Part model, mm, in its own coordinate system. Give positions to 0.01 mm unless a question says otherwise; leave off trailing zeros. Write each loop counter-clockwise with the first axis right and the second up, starting at its lowest first coordinate (ties: lowest second). Pieces come first, ordered by that corner, then holes. Notation, with made-up numbers: (80, 53) - (109, 53) arc R10 ccw to (109, 61) - close; hole circle Ø1 at (53.25, 29.25). An arc over 180 degrees is marked (long way). Answer as a JSON object with one key per item and string values. Group by question number.
```python
from build123d import *

# Parameters (mm, degrees)
BOSS_EXTRUDE1_DEPTH          = 3
MOUNTING_SLOTS_REACH         = 173.039
SKETCH2_W                    = 3.2
SKETCH2_H                    = 15
CASTER_AND_WHEEL_SLOTS_REACH = 173.039
SKETCH3_R                    = 4.7
SKETCH3_W                    = 12
SKETCH3_H                    = 68


with BuildPart() as part:
    # Sketch1 → Boss-Extrude1 (new body)
    with BuildSketch(Plane.XY):
        with BuildLine():
            Line((-107.5, -45.307284183), (-107.5, 47.371965948))
            ThreePointArc((-107.5, 47.371965948), (-94.261836832, 91.449819149), (-58.928571429, 120.939927031))
            ThreePointArc((-58.928571429, 120.939927031), (0, 133), (58.928571429, 120.939927031))
            ThreePointArc((58.928571429, 120.939927031), (94.261836832, 91.449819149), (107.5, 47.371965948))
            Line((107.5, 47.371965948), (107.5, -45.307284183))
            ThreePointArc((107.5, -45.307284183), (97.216406667, -84.545309636), (69.009433962, -113.695637666))
            ThreePointArc((69.009433962, -113.695637666), (0, -133), (-69.009433962, -113.695637666))
            ThreePointArc((-69.009433962, -113.695637666), (-97.216406667, -84.545309636), (-107.5, -45.307284183))
        make_face()
    extrude(amount=BOSS_EXTRUDE1_DEPTH)

    # Sketch2 → mounting slots (cut, up to next)
    with BuildSketch(Plane.XY.offset(3), mode=Mode.PRIVATE) as mounting_slots_sk1:
        with Locations((98.1, -52.5)):
            Rectangle(SKETCH2_W, SKETCH2_H)
    mounting_slots_tool1 = extrude(mounting_slots_sk1.sketch, amount=-MOUNTING_SLOTS_REACH, mode=Mode.PRIVATE) & part.part
    # Sketch2 → mounting slots (cut, up to next)
    with BuildSketch(Plane.XY.offset(3), mode=Mode.PRIVATE) as mounting_slots_sk2:
        with Locations((98.1, 52.5)):
            Rectangle(SKETCH2_W, SKETCH2_H)
    mounting_slots_tool2 = extrude(mounting_slots_sk2.sketch, amount=-MOUNTING_SLOTS_REACH, mode=Mode.PRIVATE) & part.part
    # Sketch2 → mounting slots (cut, up to next)
    with BuildSketch(Plane.XY.offset(3), mode=Mode.PRIVATE) as mounting_slots_sk3:
        with Locations((-98.1, 52.5)):
            Rectangle(SKETCH2_W, SKETCH2_H)
    mounting_slots_tool3 = extrude(mounting_slots_sk3.sketch, amount=-MOUNTING_SLOTS_REACH, mode=Mode.PRIVATE) & part.part
    # Sketch2 → mounting slots (cut, up to next)
    with BuildSketch(Plane.XY.offset(3), mode=Mode.PRIVATE) as mounting_slots_sk4:
        with Locations((-98.1, -52.5)):
            Rectangle(SKETCH2_W, SKETCH2_H)
    mounting_slots_tool4 = extrude(mounting_slots_sk4.sketch, amount=-MOUNTING_SLOTS_REACH, mode=Mode.PRIVATE) & part.part
    # Sketch2 → mounting slots (cut, up to next)
    with BuildSketch(Plane.XY.offset(3), mode=Mode.PRIVATE) as mounting_slots_sk5:
        with Locations((52.79, 97.254160418)):
            Rectangle(SKETCH2_W, SKETCH2_H)
    mounting_slots_tool5 = extrude(mounting_slots_sk5.sketch, amount=-MOUNTING_SLOTS_REACH, mode=Mode.PRIVATE) & part.part
    # Sketch2 → mounting slots (cut, up to next)
    with BuildSketch(Plane.XY.offset(3), mode=Mode.PRIVATE) as mounting_slots_sk6:
        with Locations((52.79, -97.254160418)):
            Rectangle(SKETCH2_W, SKETCH2_H)
    mounting_slots_tool6 = extrude(mounting_slots_sk6.sketch, amount=-MOUNTING_SLOTS_REACH, mode=Mode.PRIVATE) & part.part
    # Sketch2 → mounting slots (cut, up to next)
    with BuildSketch(Plane.XY.offset(3), mode=Mode.PRIVATE) as mounting_slots_sk7:
        with Locations((-52.79, 97.254160418)):
            Rectangle(SKETCH2_W, SKETCH2_H)
    mounting_slots_tool7 = extrude(mounting_slots_sk7.sketch, amount=-MOUNTING_SLOTS_REACH, mode=Mode.PRIVATE) & part.part
    # Sketch2 → mounting slots (cut, up to next)
    with BuildSketch(Plane.XY.offset(3), mode=Mode.PRIVATE) as mounting_slots_sk8:
        with Locations((-52.79, -97.254160418)):
            Rectangle(SKETCH2_W, SKETCH2_H)
    mounting_slots_tool8 = extrude(mounting_slots_sk8.sketch, amount=-MOUNTING_SLOTS_REACH, mode=Mode.PRIVATE) & part.part
    # Sketch2 → mounting slots (cut, up to next)
    with BuildSketch(Plane.XY.offset(3), mode=Mode.PRIVATE) as mounting_slots_sk9:
        with BuildLine():
            Line((31.1, -18.6), (61.1, -18.6))
            Line((61.1, -18.6), (61.1, -15.1))
            Line((61.1, -15.1), (53.5, -15.1))
            Line((53.5, -15.1), (53, -13.6))
            Line((53, -13.6), (53.5, -13.6))
            Line((53.5, -13.6), (53.5, -10.5))
            Line((53.5, -10.5), (40.7, -10.5))
            Line((40.7, -10.5), (40.7, -7.6))
            ThreePointArc((40.7, -7.6), (39.7, -6.6), (38.7, -7.6))
            Line((38.7, -7.6), (38.7, -10.5))
            Line((38.7, -10.5), (38.9, -13.6))
            Line((38.9, -13.6), (39.4, -13.6))
            Line((39.4, -13.6), (38.9, -15.1))
            Line((38.9, -15.1), (36.2, -15.1))
            Line((36.2, -15.1), (36.2, -7.6))
            ThreePointArc((36.2, -7.6), (35.2, -6.6), (34.2, -7.6))
            Line((34.2, -7.6), (34.2, -15.1))
            Line((34.2, -15.1), (31.1, -15.1))
            Line((31.1, -15.1), (31.1, -18.6))
        make_face()
    mounting_slots_tool9 = extrude(mounting_slots_sk9.sketch, amount=-MOUNTING_SLOTS_REACH, mode=Mode.PRIVATE) & part.part
    # Sketch2 → mounting slots (cut, up to next)
    with BuildSketch(Plane.XY.offset(3), mode=Mode.PRIVATE) as mounting_slots_sk10:
        with BuildLine():
            Line((31.1, 5.4), (61.1, 5.4))
            Line((61.1, 5.4), (61.1, 8.9))
            Line((61.1, 8.9), (53.5, 8.9))
            Line((53.5, 8.9), (53, 10.4))
            Line((53, 10.4), (53.5, 10.4))
            Line((53.5, 10.4), (53.5, 13.5))
            Line((53.5, 13.5), (40.7, 13.5))
            Line((40.7, 13.5), (40.7, 16.4))
            ThreePointArc((40.7, 16.4), (39.7, 17.4), (38.7, 16.4))
            Line((38.7, 16.4), (38.7, 13.5))
            Line((38.7, 13.5), (38.9, 10.4))
            Line((38.9, 10.4), (39.4, 10.4))
            Line((39.4, 10.4), (38.9, 8.9))
            Line((38.9, 8.9), (36.2, 8.9))
            Line((36.2, 8.9), (36.2, 16.4))
            ThreePointArc((36.2, 16.4), (35.2, 17.4), (34.2, 16.4))
            Line((34.2, 16.4), (34.2, 8.9))
            Line((34.2, 8.9), (31.1, 8.9))
            Line((31.1, 8.9), (31.1, 5.4))
        make_face()
    mounting_slots_tool10 = extrude(mounting_slots_sk10.sketch, amount=-MOUNTING_SLOTS_REACH, mode=Mode.PRIVATE) & part.part
    # Sketch2 → mounting slots (cut, up to next)
    with BuildSketch(Plane.XY.offset(3), mode=Mode.PRIVATE) as mounting_slots_sk11:
        with BuildLine():
            Line((-60.9, -18.6), (-30.9, -18.6))
            Line((-30.9, -18.6), (-30.9, -15.1))
            Line((-30.9, -15.1), (-38.5, -15.1))
            Line((-38.5, -15.1), (-39, -13.6))
            Line((-39, -13.6), (-38.5, -13.6))
            Line((-38.5, -13.6), (-38.5, -10.5))
            Line((-38.5, -10.5), (-51.3, -10.5))
            Line((-51.3, -10.5), (-51.3, -7.6))
            ThreePointArc((-51.3, -7.6), (-52.3, -6.6), (-53.3, -7.6))
            Line((-53.3, -7.6), (-53.3, -10.5))
            Line((-53.3, -10.5), (-53.1, -13.6))
            Line((-53.1, -13.6), (-52.6, -13.6))
            Line((-52.6, -13.6), (-53.1, -15.1))
            Line((-53.1, -15.1), (-55.8, -15.1))
            Line((-55.8, -15.1), (-55.8, -7.6))
            ThreePointArc((-55.8, -7.6), (-56.8, -6.6), (-57.8, -7.6))
            Line((-57.8, -7.6), (-57.8, -15.1))
            Line((-57.8, -15.1), (-60.9, -15.1))
            Line((-60.9, -15.1), (-60.9, -18.6))
        make_face()
    mounting_slots_tool11 = extrude(mounting_slots_sk11.sketch, amount=-MOUNTING_SLOTS_REACH, mode=Mode.PRIVATE) & part.part
    # Sketch2 → mounting slots (cut, up to next)
    with BuildSketch(Plane.XY.offset(3), mode=Mode.PRIVATE) as mounting_slots_sk12:
        with BuildLine():
            Line((-60.9, 5.4), (-30.9, 5.4))
            Line((-30.9, 5.4), (-30.9, 8.9))
            Line((-30.9, 8.9), (-38.5, 8.9))
            Line((-38.5, 8.9), (-39, 10.4))
            Line((-39, 10.4), (-38.5, 10.4))
            Line((-38.5, 10.4), (-38.5, 13.5))
            Line((-38.5, 13.5), (-51.3, 13.5))
            Line((-51.3, 13.5), (-51.3, 16.4))
            ThreePointArc((-51.3, 16.4), (-52.3, 17.4), (-53.3, 16.4))
            Line((-53.3, 16.4), (-53.3, 13.5))
            Line((-53.3, 13.5), (-53.1, 10.4))
            Line((-53.1, 10.4), (-52.6, 10.4))
            Line((-52.6, 10.4), (-53.1, 8.9))
            Line((-53.1, 8.9), (-55.8, 8.9))
            Line((-55.8, 8.9), (-55.8, 16.4))
            ThreePointArc((-55.8, 16.4), (-56.8, 17.4), (-57.8, 16.4))
            Line((-57.8, 16.4), (-57.8, 8.9))
            Line((-57.8, 8.9), (-60.9, 8.9))
            Line((-60.9, 8.9), (-60.9, 5.4))
        make_face()
    mounting_slots_tool12 = extrude(mounting_slots_sk12.sketch, amount=-MOUNTING_SLOTS_REACH, mode=Mode.PRIVATE) & part.part
    add(mounting_slots_tool1.solids().sort_by_distance((98.1, -52.5, 3))[0], mode=Mode.SUBTRACT)
    add(mounting_slots_tool2.solids().sort_by_distance((98.1, 52.5, 3))[0], mode=Mode.SUBTRACT)
    add(mounting_slots_tool3.solids().sort_by_distance((-98.1, 52.5, 3))[0], mode=Mode.SUBTRACT)
    add(mounting_slots_tool4.solids().sort_by_distance((-98.1, -52.5, 3))[0], mode=Mode.SUBTRACT)
    add(mounting_slots_tool5.solids().sort_by_distance((52.79, 97.25416, 3))[0], mode=Mode.SUBTRACT)
    add(mounting_slots_tool6.solids().sort_by_distance((52.79, -97.25416, 3))[0], mode=Mode.SUBTRACT)
    add(mounting_slots_tool7.solids().sort_by_distance((-52.79, 97.25416, 3))[0], mode=Mode.SUBTRACT)
    add(mounting_slots_tool8.solids().sort_by_distance((-52.79, -97.25416, 3))[0], mode=Mode.SUBTRACT)
    add(mounting_slots_tool9.solids().sort_by_distance((44.9582, -14.653776, 3))[0], mode=Mode.SUBTRACT)
    add(mounting_slots_tool10.solids().sort_by_distance((44.9582, 9.346224, 3))[0], mode=Mode.SUBTRACT)
    add(mounting_slots_tool11.solids().sort_by_distance((-47.0418, -14.653776, 3))[0], mode=Mode.SUBTRACT)
    add(mounting_slots_tool12.solids().sort_by_distance((-47.0418, 9.346224, 3))[0], mode=Mode.SUBTRACT)

    # Sketch3 → caster and wheel slots (cut, up to next)
    with BuildSketch(Plane.XY.offset(3), mode=Mode.PRIVATE) as caster_and_wheel_slots_sk1:
        with Locations((0, 118)):
            Circle(SKETCH3_R)
    caster_and_wheel_slots_tool1 = extrude(caster_and_wheel_slots_sk1.sketch, amount=-CASTER_AND_WHEEL_SLOTS_REACH, mode=Mode.PRIVATE) & part.part
    # Sketch3 → caster and wheel slots (cut, up to next)
    with BuildSketch(Plane.XY.offset(3), mode=Mode.PRIVATE) as caster_and_wheel_slots_sk2:
        with Locations((75, -46)):
            Rectangle(SKETCH3_W, SKETCH3_H)
    caster_and_wheel_slots_tool2 = extrude(caster_and_wheel_slots_sk2.sketch, amount=-CASTER_AND_WHEEL_SLOTS_REACH, mode=Mode.PRIVATE) & part.part
    # Sketch3 → caster and wheel slots (cut, up to next)
    with BuildSketch(Plane.XY.offset(3), mode=Mode.PRIVATE) as caster_and_wheel_slots_sk3:
        with Locations((-75, -46)):
            Rectangle(SKETCH3_W, SKETCH3_H)
    caster_and_wheel_slots_tool3 = extrude(caster_and_wheel_slots_sk3.sketch, amount=-CASTER_AND_WHEEL_SLOTS_REACH, mode=Mode.PRIVATE) & part.part
    add(caster_and_wheel_slots_tool1.solids().sort_by_distance((0, 118, 3))[0], mode=Mode.SUBTRACT)
    add(caster_and_wheel_slots_tool2.solids().sort_by_distance((75, -46, 3))[0], mode=Mode.SUBTRACT)
    add(caster_and_wheel_slots_tool3.solids().sort_by_distance((-75, -46, 3))[0], mode=Mode.SUBTRACT)


solid = part.part
```
1) Drop flat-ended pins along their axis: P1, Ø1.5, axis at y = -98.5, z = 1.5, coming from the -X side; P2, Ø0.9, axis at x = 58.5, z = 1.5, coming from the -Y side; P3, Ø0.9, axis at x = -59, z = 2, coming from the -Y side. Give the stop position or say it passes through.
2) Band-saw the part on D-D (x = -84). List the corners of the cut face in (y, z).
3) Mould opens along Y. For faces 1 (the cylindrical face through (-94.62, 90.9, 1.48)), 2 (the cylindrical face through (-0.61, 122.66, 1.52)), 3 (the cylindrical face through (-96.933, -85.045, 1.479)) say: pulls with the +Y half, pulls with the -Y half, needs draft (parallel to the pull), parting line crosses it, or undercut.
4) Band-saw the part on C-C (z = 2.3). State how many separate pieces and enclosed holes the cut face has, plus the area to 3 significant figures.
5) Probe line 1 (X direction, y = -39.5, z = 2); line 2 (X direction, y = -16, z = 1.15); line 3 (X direction, y = -7, z = 0.95). List the from-to ranges inside material, lowest first.
6) Band-saw the part on B-B (x = 75). List the corners of the cut face in (y, z).
7) Band-saw the part on A-A (x = 0). List the corners of the cut face in (y, z), plus the area to 3 significant figures.
Verdict:
{
 "1": {"P1": "x = -87.91", "P2": "y = -119.66", "P3": "y = -119.42"},
 "2": {"outline": "(-101.94, 0) - (104.01, 0) - (104.01, 3) - (-101.94, 3) - close"},
 "3": {"face 1": "pulls with the +Y half", "face 2": "undercut", "face 3": "pulls with the -Y half"},
 "4": {"separate pieces": "1", "enclosed holes": "15", "area": "46,800 mm2"},
 "5": {"line 1": "-107.5 to -81, -69 to 69, 81 to 107.5", "line 2": "-107.5 to -81, -69 to -60.9, -30.9 to 31.1, 61.1 to 69, 81 to 107.5", "line 3": "-107.5 to -57.6, -56 to -53.1, -51.5 to 34.4, 36 to 38.9, 40.5 to 107.5"},
 "6": {"outline": "(-109.68, 0) - (-80, 0) - (-80, 3) - (-109.68, 3) - close; (-12, 0) - (111.74, 0) - (111.74, 3) - (-12, 3) - close"},
 "7": {"outline": "(-133, 0) - (113.3, 0) - (113.3, 3) - (-133, 3) - close; (122.7, 0) - (133, 0) - (133, 3) - (122.7, 3) - close", "area": "770 mm2"}
}
